Verification items for the finished model (mm, model axes). A direction names the side the tool comes from. Coordinates: 2 decimals unless noted, no trailing zeros. Order: outer loops, then holes, each group sorted by start corner. A loop starts at its lowest first (then second) coordinate and runs counter-clockwise, first axis right, second up. Notation, with made-up numbers: M 39,54.25 L 78,54.25 A25 cw 78,90.25 Z; hole C -2,-4.5 d11. An arc over 180 degrees is marked long. Answer as a JSON object with one key per item and string values. Group by question number.
(1) Access from +Z, -Z, +X, -X, +Y, -Y to the whole of each face (thin tool, end or side, straight path). Record for faces 5 (the face through (1.27, -0.97, 1.48)), 6 (the face through (-0.94, -1.5, 7.68)), 7 (the face through (0, -2.75, 4)).
(2) Material ranges on line 1 (Y direction, x = 1.75, z = 6.25); line 2 (Y direction, x = -3, z = 4.5); line 3 (Z direction, x = 0, y = 3.6), recorded low to high.
(3) Mould release check, pull along Z, two halves, no side actions. Record for faces 1 (the face through (-0.94, 1.5, 7.68)), 2 (the face through (0, 2.75, 4)), 3 (the face through (-0.06, 4.48, 1.31)), 4 (the face through (-2.859, -3.226, 11.797)): released by +Z, released by -Z, zero draft, split by the parting line, or undercut.
(4) Cross-section at B-B (x = 1.25). Enter the section's corners in (y, z), plus the area to 3 significant figures.
(5) Cross-section at A-A (z = 4.25). Enter the section's corners in (x, y), plus the area to 3 significant figures.
(6) Cross-section at D-D (z = 8). Enter the section's corners in (x, y).
(7) Cross-section at C-C (y = 0.25). Enter the section's corners in (x, z), plus the area to 3 significant figures.
from build123d import *

# Parameters (mm, degrees)
SKETCH1_W           = 8
SKETCH1_H           = 10
BOSS_EXTRUDE1_DEPTH = 3
SKETCH2_W           = 8
SKETCH2_H           = 3.5
BOSS_EXTRUDE2_DEPTH = 10
CUT_EXTRUDE1_START  = -8
SKETCH3_W           = 2.7
SKETCH3_H           = 5.5
CUT_EXTRUDE1_DEPTH  = 8
CUT_EXTRUDE2_REACH  = 16.491
SKETCH4_R           = 1.6
SKETCH5_R           = 1.75
CUT_EXTRUDE3_DEPTH  = 17.881943016
FILLET1_R           = 4
FILLET2_START       = -5
FILLET2_DEPTH       = 10
FILLET2_2_DEPTH     = 10


with BuildPart() as part:
    # Sketch1 → Boss-Extrude1 (new body)
    with BuildSketch(Plane.XY):
        Rectangle(SKETCH1_W, SKETCH1_H)
    extrude(amount=BOSS_EXTRUDE1_DEPTH)

    # Sketch2 → Boss-Extrude2 (add)
    with BuildSketch(Plane.XY.offset(3)):
        with Locations((0, 3.25)):
            Rectangle(SKETCH2_W, SKETCH2_H)
        with Locations((0, -3.25)):
            Rectangle(SKETCH2_W, SKETCH2_H)
    extrude(amount=BOSS_EXTRUDE2_DEPTH)

    # Sketch3 → Cut-Extrude1 (cut)
    with BuildSketch(Plane(origin=(4, 0, 0), x_dir=(0, 0, -1), z_dir=(1, 0, 0)).offset(CUT_EXTRUDE1_START)):
        with Locations((-4.35, 0)):
            Rectangle(SKETCH3_W, SKETCH3_H)
    extrude(amount=CUT_EXTRUDE1_DEPTH, mode=Mode.SUBTRACT)

    # Sketch4 → Cut-Extrude2 (cut, up to next)
    with BuildSketch(Plane(origin=(0, 0, 0), x_dir=(-1, 0, 0), z_dir=(0, 0, -1)), mode=Mode.PRIVATE) as cut_extrude2_sk1:
        Circle(SKETCH4_R)
    cut_extrude2_tool1 = extrude(cut_extrude2_sk1.sketch, amount=-CUT_EXTRUDE2_REACH, mode=Mode.PRIVATE) & part.part
    add(cut_extrude2_tool1.solids().sort_by_distance((0, 0, 0))[0], mode=Mode.SUBTRACT)

    # Sketch5 → Cut-Extrude3 (cut, through all)
    with BuildSketch(Plane(origin=(0, 5, 0), x_dir=(1, 0, 0), z_dir=(0, 1, 0))):
        with Locations(Location((0, -9.35, 0), (0, 0, 180))):
            Circle(SKETCH5_R)
    extrude(amount=-CUT_EXTRUDE3_DEPTH, mode=Mode.SUBTRACT)

    # Fillet1
    fillet1_edges = [part.edges().sort_by_distance(p)[0] for p in [
        (-4, -3.25, 13),
        (-4, 3.25, 13),
        (4, -3.25, 13),
        (4, 3.25, 13),
    ]]
    fillet(fillet1_edges, radius=FILLET1_R - 0.0001)  # a hair under: the kernel refuses the full size

    # Fillet2: read off the stored shape, not the designer's step
    # Fillet2 outline → Fillet2 (cut)
    with BuildSketch(Plane(origin=(0, 0, 0), x_dir=(1, 0, 0), z_dir=(0, 1, 0)).offset(FILLET2_START)):
        with BuildLine():
            ThreePointArc((-4, -3), (-3.121320344, -0.878679656), (-1, 0))
            Line((-1, 0), (-4, 0))
            Line((-4, 0), (-4, -3))
        make_face()
        with BuildLine():
            ThreePointArc((1, 0), (3.121320344, -0.878679656), (4, -3))
            Line((4, -3), (4, 0))
            Line((4, 0), (1, 0))
        make_face()
    extrude(amount=FILLET2_DEPTH, mode=Mode.SUBTRACT)

    # Fillet2 2 outline → Fillet2 2 (cut)
    with BuildSketch(Plane.YZ.offset(FILLET2_START)):
        with BuildLine():
            Line((5, 0), (5, 3))
            ThreePointArc((5, 3), (4.121320344, 0.878679656), (2, 0))
            Line((2, 0), (5, 0))
        make_face()
        with BuildLine():
            ThreePointArc((-2, 0), (-4.121320344, 0.878679656), (-5, 3))
            Line((-5, 3), (-5, 0))
            Line((-5, 0), (-2, 0))
        make_face()
    extrude(amount=FILLET2_2_DEPTH, mode=Mode.SUBTRACT)


solid = part.part
Taken from the geometry:
{
 "1": {"face 5": "-Z", "face 6": "+Z, +X, -X", "face 7": "+X, -X"},
 "2": {"line 1": "y = -5 to -1.5, 1.5 to 5", "line 2": "y = -5 to -2.75, 2.75 to 5", "line 3": "z = 0.46 to 7.6, 11.1 to 13"},
 "3": {"face 1": "zero draft", "face 2": "undercut", "face 3": "released by -Z", "face 4": "released by +Z"},
 "4": {"outline": "M -5,3 A3 ccw -2.25,0.01 L -1,0.01 L -1,3 L -2.75,3 L -2.75,5.7 L -1.5,5.7 L -1.5,8.13 L -5,8.13 Z; M -5,10.57 L -1.5,10.57 L -1.5,12.8 L -5,12.8 Z; M 1,0.01 L 2.25,0.01 A3 ccw 5,3 L 5,8.13 L 1.5,8.13 L 1.5,5.7 L 2.75,5.7 L 2.75,3 L 1,3 Z; M 1.5,10.57 L 5,10.57 L 5,12.8 L 1.5,12.8 Z", "area": "64.8 mm²"},
 "5": {"outline": "M -4,-5 L 4,-5 L 4,-2.75 L -4,-2.75 Z; M -4,2.75 L 4,2.75 L 4,5 L -4,5 Z", "area": "36.0 mm²"},
 "6": {"outline": "M -4,-5 L -1.11,-5 L -1.11,-1.5 L -4,-1.5 Z; M -4,1.5 L -1.11,1.5 L -1.11,5 L -4,5 Z; M 1.11,-5 L 4,-5 L 4,-1.5 L 1.11,-1.5 Z; M 1.11,1.5 L 4,1.5 L 4,5 L 1.11,5 Z"},
 "7": {"outline": "M -4,3 A3 ccw -1.58,0.06 L -1.58,3 Z; M 1.58,0.06 A3 ccw 4,3 L 1.58,3 Z", "area": "10.7 mm²"}
}
